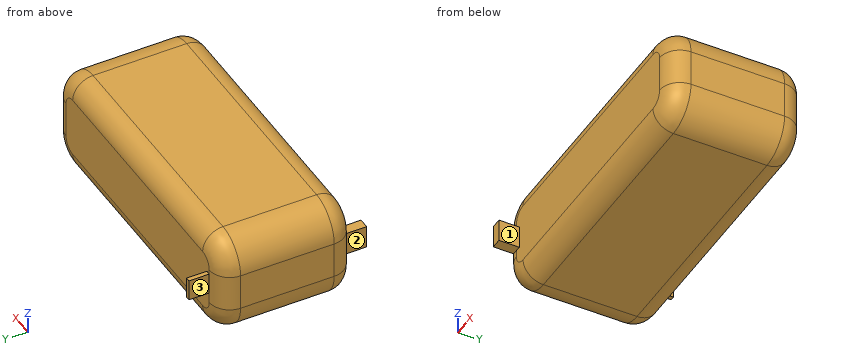
```python
from build123d import *

# Parameters (mm, degrees)
SKETCH1_W           = 75
SKETCH1_H           = 33
BOSS_EXTRUDE1_DEPTH = 25
FILLET1_R           = 5
FILLET2_R           = 8
SKETCH2_W           = 2.553418492
SKETCH2_H           = 5.632377872
BOSS_EXTRUDE2_DEPTH = 5
SKETCH3_W           = 1.096638537
SKETCH3_H           = 5.251652717
BOSS_EXTRUDE3_DEPTH = 5


with BuildPart() as part:
    # Sketch1 → Boss-Extrude1 (new body)
    with BuildSketch(Plane.XY):
        Rectangle(SKETCH1_W, SKETCH1_H)
    extrude(amount=BOSS_EXTRUDE1_DEPTH)

    # Fillet1
    fillet1_edges = [part.edges().sort_by_distance(p)[0] for p in [
        (0, -16.5, 25),
        (0, -16.5, 0),
        (0, 16.5, 0),
        (0, 16.5, 25),
        (37.5, -16.5, 12.5),
        (-37.5, -16.5, 12.5),
        (-37.5, 16.5, 12.5),
        (37.5, 16.5, 12.5),
    ]]
    fillet(fillet1_edges, radius=FILLET1_R)

    # Fillet2
    # the kernel refuses this fillet: 8 mm, written as the material it takes off along each edge
    with BuildSketch(Plane(origin=(-29.5, 16.5, 17), x_dir=(-1, 0, 0), z_dir=(0, 0, -1))) as fillet2_piece_1:
        with BuildLine():
            CenterArc((3, -5), 5, 0, 90)
            Line((8, -5), (8, 0))
            Line((8, 0), (3, 0))
        make_face()
    revolve(axis=Axis((-29.5, 16.5, 17), (0, 1, 0)), revolution_arc=90, mode=Mode.SUBTRACT)
    with BuildSketch(Plane(origin=(-29.5, 16.5, 8), x_dir=(0, 0, -1), z_dir=(1, 0, 0))) as fillet2_piece_2:
        with BuildLine():
            CenterArc((3, -5), 5, 0, 90)
            Line((8, -5), (8, 0))
            Line((8, 0), (3, 0))
        make_face()
    revolve(axis=Axis((-29.5, 16.5, 8), (0, 1, 0)), revolution_arc=90, mode=Mode.SUBTRACT)
    with BuildSketch(Plane(origin=(29.5, 16.5, 17), x_dir=(0, 0, 1), z_dir=(-1, 0, 0))) as fillet2_piece_3:
        with BuildLine():
            CenterArc((3, -5), 5, 0, 90)
            Line((8, -5), (8, 0))
            Line((8, 0), (3, 0))
        make_face()
    revolve(axis=Axis((29.5, 16.5, 17), (0, 1, 0)), revolution_arc=90, mode=Mode.SUBTRACT)
    with BuildSketch(Plane(origin=(29.5, 16.5, 8), x_dir=(1, 0, 0), z_dir=(0, 0, 1))) as fillet2_piece_4:
        with BuildLine():
            CenterArc((3, -5), 5, 0, 90)
            Line((8, -5), (8, 0))
            Line((8, 0), (3, 0))
        make_face()
    revolve(axis=Axis((29.5, 16.5, 8), (0, 1, 0)), revolution_arc=90, mode=Mode.SUBTRACT)
    with BuildSketch(Plane(origin=(-29.5, -16.5, 17), x_dir=(0, 0, 1), z_dir=(1, 0, 0))) as fillet2_piece_5:
        with BuildLine():
            CenterArc((3, -5), 5, 0, 90)
            Line((8, -5), (8, 0))
            Line((8, 0), (3, 0))
        make_face()
    revolve(axis=Axis((-29.5, -16.5, 17), (0, -1, 0)), revolution_arc=90, mode=Mode.SUBTRACT)
    with BuildSketch(Plane(origin=(-29.5, -16.5, 8), x_dir=(-1, 0, 0), z_dir=(0, 0, 1))) as fillet2_piece_6:
        with BuildLine():
            CenterArc((3, -5), 5, 0, 90)
            Line((8, -5), (8, 0))
            Line((8, 0), (3, 0))
        make_face()
    revolve(axis=Axis((-29.5, -16.5, 8), (0, -1, 0)), revolution_arc=90, mode=Mode.SUBTRACT)
    with BuildSketch(Plane(origin=(29.5, -16.5, 17), x_dir=(1, 0, 0), z_dir=(0, 0, -1))) as fillet2_piece_7:
        with BuildLine():
            CenterArc((3, -5), 5, 0, 90)
            Line((8, -5), (8, 0))
            Line((8, 0), (3, 0))
        make_face()
    revolve(axis=Axis((29.5, -16.5, 17), (0, -1, 0)), revolution_arc=90, mode=Mode.SUBTRACT)
    with BuildSketch(Plane(origin=(29.5, -16.5, 8), x_dir=(0, 0, -1), z_dir=(-1, 0, 0))) as fillet2_piece_8:
        with BuildLine():
            CenterArc((3, -5), 5, 0, 90)
            Line((8, -5), (8, 0))
            Line((8, 0), (3, 0))
        make_face()
    revolve(axis=Axis((29.5, -16.5, 8), (0, -1, 0)), revolution_arc=90, mode=Mode.SUBTRACT)
    with BuildSketch(Plane(origin=(37.5, -16.5, 0), x_dir=(0, 0, 1), z_dir=(0, 1, 0)), Plane(origin=(37.5, -16.5, 25), x_dir=(-1, 0, 0), z_dir=(0, 1, 0)), Plane(origin=(-37.5, 16.5, 0), x_dir=(0, 0, 1), z_dir=(0, -1, 0)), Plane(origin=(-37.5, 16.5, 25), x_dir=(1, 0, 0), z_dir=(0, -1, 0))) as fillet2_piece_9:
        with BuildLine():
            CenterArc((FILLET2_R, -FILLET2_R), FILLET2_R, 90, 90)
            Line((0, -FILLET2_R), (0, 0))
            Line((0, 0), (FILLET2_R, 0))
        make_face()
    extrude(amount=33, mode=Mode.SUBTRACT)

    # Sketch2 → Boss-Extrude2 (add)
    with BuildSketch(Plane.XZ.offset(16.5)):
        with Locations((-32.5, 12.5)):
            Rectangle(SKETCH2_W, SKETCH2_H)
    extrude(amount=BOSS_EXTRUDE2_DEPTH)

    # Sketch3 → Boss-Extrude3 (add)
    with BuildSketch(Plane(origin=(0, 16.5, 0), x_dir=(1, 0, 0), z_dir=(0, 1, 0))):
        with Locations((-31.951680732, -13.240900807)):
            Rectangle(SKETCH3_W, SKETCH3_H)
    extrude(amount=BOSS_EXTRUDE3_DEPTH)


solid = part.part
```
Read the model definition and answer for the solid it produces. Units are mm, in the model's axes. Face numbers are marked on the shaded views. A direction names the side the tool comes from. Give positions to 0.01 mm unless a question says otherwise; leave off trailing zeros. Loops run counter-clockwise (first coordinate to the right, second up) from the corner with the lowest first, then second, coordinate; pieces in that order, holes last.
Item 1: The part is cut by section C-C (y = 18). Write down the section's boundary in (x, z).
Item 2: The part is cut by section A-A (x = -8). Write down the section's boundary in (y, z).
Item 3: For the marked faces 1, 2 and 3, determine the directions among +Z, -Z, +X, -X, +Y, -Y from which every point of the face is accessible in a straight line to the end or side of a thin tool.
Item 4: Find the intervals of material crossed by line 1 along Y through (x, z) = (-15, 19.75); line 2 along X through (y, z) = (-17, 12.5); line 3 along Y through (x, z) = (-30.5, 2), in increasing order.
Item 5: The part is cut by section B-B (y = 5.5). Write down the section's boundary in (x, z), and give its area (3 significant figures).
Item 6: Each of these flat-tipped pins is pushed along its axis until it touches: pin 1 Ø1.5 at (x, z) = (-22, 10) entering from -Y; pin 2 Ø1.5 at (y, z) = (19.5, 12.5) entering from +X; pin 3 Ø0.8 at (x, y) = (-32.5, -18) entering from +Z. Where does it stop, or does it pass through?
Taken from the geometry:
1. outline: (-32.5, 10.62) - (-31.4, 10.62) - (-31.4, 15.87) - (-32.5, 15.87) - close
2. outline: (-16.5, 5) arc R5 ccw to (-11.5, 0) - (11.5, 0) arc R5 ccw to (16.5, 5) - (16.5, 20) arc R5 ccw to (11.5, 25) - (-11.5, 25) arc R5 ccw to (-16.5, 20) - close
3. face 1: +Z, -Z, +X, -Y
3. face 2: +Z, -Z, -X, -Y
3. face 3: +Z, -Z, -X, +Y
4. line 1: y = -16.5 to 16.5
4. line 2: x = -33.78 to -31.22
4. line 3: y = -15.44 to 15.44
5. outline: (-37.5, 8) arc R8 ccw to (-29.5, 0) - (29.5, 0) arc R8 ccw to (37.5, 8) - (37.5, 17) arc R8 ccw to (29.5, 25) - (-29.5, 25) arc R8 ccw to (-37.5, 17) - close
5. area: 1,820 mm2
6. pin 1: stops at y = -16.5
6. pin 2: stops at x = -31.4
6. pin 3: stops at z = 15.32
